Could you check a few things on this model? Use its own coordinates, in mm. Face numbers are marked on the shaded views. A direction names the side the tool comes from. Coordinates: 2 decimals unless noted, no trailing zeros. Loops run counter-clockwise (first coordinate to the right, second up) from the corner with the lowest first, then second, coordinate; pieces in that order, holes last.
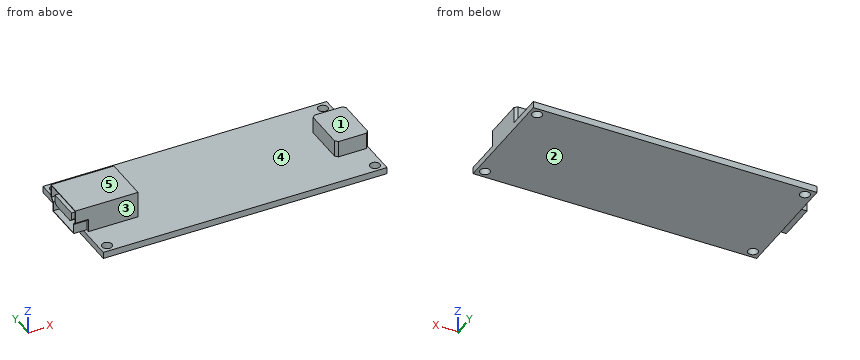
from build123d import *

# Parameters (mm, degrees)
F0_W     = 8
F0_H     = 7
F0_R     = 0.75
F0_W_2   = 5
F1_DEPTH = 1
F0_W_3   = 1.5
F2_DEPTH = 4
F3_DEPTH = 2.5
F4_W     = 4.784234
F4_H     = 1.5
F5_DEPTH = 5
F6_DEPTH = 2
F7_SIZE  = 0.4
F8_SIZE  = 0.4


with BuildPart() as f1:
    # F0 (on Top) → F1 (new body)
    with BuildSketch(Plane.XY):
        with Locations((-17.5, 0)):
            Rectangle(F0_W, F0_H)
        Polygon((21.5, 3.5), (21.5, 8.75), (-21.5, 8.75), (-21.5, 3.5), (-13.5, 3.5), (-13.5, -3.5), (-21.5, -3.5), (-21.5, -8.75), (21.5, -8.75), (21.5, -3.5), (16.5, -3.5), (16.5, 3.5), align=None)
        with Locations((-20.3, -7.55)):
            Circle(F0_R, mode=Mode.SUBTRACT)
        with Locations((20.3, -7.55)):
            Circle(F0_R, mode=Mode.SUBTRACT)
        with Locations((-20.3, 7.55)):
            Circle(F0_R, mode=Mode.SUBTRACT)
        with Locations((20.3, 7.55)):
            Circle(F0_R, mode=Mode.SUBTRACT)
        with Locations((19, 0)):
            Rectangle(F0_W_2, F0_H)
    extrude(amount=-F1_DEPTH)

    # F0 (on Top) → F2 (join)
    with BuildSketch(Plane.XY):
        with Locations((-22.25, 0)):
            Rectangle(F0_W_3, F0_H)
        with Locations((-17.5, 0)):
            Rectangle(F0_W, F0_H)
    extrude(amount=F2_DEPTH)

    # F0 (on Top) → F3 (join)
    with BuildSketch(Plane.XY):
        with Locations((19, 0)):
            Rectangle(F0_W_2, F0_H)
    extrude(amount=F3_DEPTH)

    # F4 (on face) → F5 (cut)
    with BuildSketch(Plane(origin=(-23, 0, 0), x_dir=(0, -1, 0), z_dir=(-1, 0, 0))):
        Polygon((3.4, 3.9), (-3.4, 3.9), (-3.4, 2.041421), (-2.9, 1.541421), (-2.9, 0.1), (2.9, 0.1), (2.9, 1.541421), (3.4, 2.041421), align=None)
        with Locations((0, 2.25)):
            Rectangle(F4_W, F4_H, mode=Mode.SUBTRACT)
    extrude(amount=-F5_DEPTH, mode=Mode.SUBTRACT)

    # F4 (on face) → F6 (cut)
    with BuildSketch(Plane(origin=(-23, 0, 0), x_dir=(0, -1, 0), z_dir=(-1, 0, 0))):
        Polygon((-3, 1.5), (-3.5, 2), (-3.5, 0), (-3, 0), align=None)
        Polygon((3, 1.5), (3, 0), (3.5, 0), (3.5, 2), align=None)
    extrude(amount=-F6_DEPTH, mode=Mode.SUBTRACT)

    # F7
    f7_edges = [f1.edges().sort_by_distance(p)[0] for p in [
        (-20.5, -2.392117, 1.5),
        (-20.5, 2.392117, 1.5),
    ]]
    chamfer(f7_edges, length=F7_SIZE)

    # F8
    f8_edges = [f1.edges().sort_by_distance(p)[0] for p in [
        (21.5, 3.5, 1.25),
        (16.5, 3.5, 1.25),
        (21.5, -3.5, 1.25),
        (16.5, -3.5, 1.25),
    ]]
    chamfer(f8_edges, length=F8_SIZE)


solid = f1.part
1) If I drill on L1, parallel to Y at x = -20.3, z = -0.35; L2, parallel to Y at x = -19.5, z = 1; L3, parallel to X at y = -0.75, z = 0.8, over which ranges is the centre line in solid material (lowest first)?
2) Will these pins go through, and if not, where does the flat tip stop? pin 1 (1.5 mm diameter, centred on x = -20, z = 3, fed in from -Y); pin 2 (1 mm diameter, centred on x = -5, y = 3, fed in from +Z); pin 3 (2.5 mm diameter, centred on x = 20, y = 0.5, fed in from +Z).
3) We'd pull the mould along X, two halves only. Please class the marked faces 4 and 5: released by +X, released by -X, zero draft, split by the parting line, or undercut.
4) Imagine slicing it at B-B on y = 7.55. List the corners of the cut face in (x, z) for me.
5) Imagine slicing it at C-C on y = -0.5. List the corners of the cut face in (x, z) for me.
6) For the marked faces 1, 2 and 3, which set-ups out of +Z, -Z, +X, -X, +Y, -Y let a thin tool reach every point of the face, with its end or its side?
7) Imagine slicing it at A-A on x = -20.3. State how many separate pieces and enclosed holes the cut face has, plus the area to 3 significant figures.
8) Imagine slicing it at D-D on x = -7.5. List the corners of the cut face in (y, z) for me.
Solved:
1. L1: y = -8.75 to -8.3, -6.8 to 6.8, 8.3 to 8.75
1. L2: y = -3.5 to -2.9, 2.9 to 3.5
1. L3: x = -18 to -13.5, 16.5 to 21.5
2. pin 1: stops at y = -3.5
2. pin 2: stops at z = 0
2. pin 3: stops at z = 2.5
3. face 4: undercut
3. face 5: zero draft
4. outline: (-21.5, -1) - (-21.05, -1) - (-21.05, 0) - (-21.5, 0) - close; (-19.55, -1) - (19.55, -1) - (19.55, 0) - (-19.55, 0) - close; (21.05, -1) - (21.5, -1) - (21.5, 0) - (21.05, 0) - close
5. outline: (-23, 0) - (-21.5, 0) - (-21.5, -1) - (21.5, -1) - (21.5, 2.5) - (16.5, 2.5) - (16.5, 0) - (-13.5, 0) - (-13.5, 4) - (-23, 4) - (-23, 3.9) - (-18, 3.9) - (-18, 3) - (-23, 3) - (-23, 1.5) - (-18, 1.5) - (-18, 0.1) - (-23, 0.1) - close
6. face 1: +Z, +X, +Y, -Y
6. face 2: -Z, +X, -X, +Y, -Y
6. face 3: +Z, +X, -X, -Y
7. separate pieces: 4
7. enclosed holes: 1
7. area: 25.4 mm2
8. outline: (-8.75, -1) - (8.75, -1) - (8.75, 0) - (-8.75, 0) - close
